The listing builds one solid part. Answer for the finished solid, in the listing's coordinates (mm). A direction names the side the tool comes from. Give positions to 0.01 mm unless a question says otherwise; leave off trailing zeros. Order: outer loops, then holes, each group sorted by start corner. A loop starts at its lowest first (then second) coordinate and runs counter-clockwise, first axis right, second up. Notation, with made-up numbers: (59.25, 3) -> (86.25, 3) arc R20 cw to (86.25, 15) -> close; hole circle Ø1 at (6, 52.25). An arc over 180 degrees is marked (long way). Write item = value, one per line. Start each with the question number.
```python
from build123d import *

# Parameters (mm, degrees)
SKETCH1_R                     = 36.6395
HOUSING_FITTING_EXTRUDE_DEPTH = 16.637
HOUSING_BODY_1_DEPTH          = 21.2725
SKETCH3_R                     = 6.731
IMPELLER_BORE_DEPTH           = 17.018
SKETCH4_R                     = 4
SHAFT_BORE_DEPTH              = 20.8915
O_RING_CUT_DEPTH              = 1.27
O_RING_CUT_DEPTH_BACK         = 3.175
SKETCH5_R                     = 36.6395
SKETCH5_R_2                   = 34.2265
SKETCH12_R                    = 3.175
CUT_EXTRUDE2_DEPTH            = 21.2725
CIRPATTERN1_COUNT             = 8
SKETCH13_R                    = 3.175
CUT_EXTRUDE3_DEPTH            = 16.51
SKETCH14_R                    = 3.175
SKETCH14_R_2                  = 3.392842108
CUT_EXTRUDE4_DEPTH            = 16.51
SKETCH15_R                    = 3.175
CUT_EXTRUDE5_DEPTH            = 10.922
FILLET1_R                     = 6.604
SKETCH17_R                    = 17.5006
CUT_EXTRUDE8_DEPTH            = 25.2095
BOSS_EXTRUDE1_START           = 6.35
SKETCH18_R                    = 17.5006
SKETCH18_R_2                  = 15.875
BOSS_EXTRUDE1_DEPTH           = 6.35


with BuildPart() as part:
    # Sketch1 → Housing Fitting Extrude (new body)
    with BuildSketch(Plane(origin=(0, 0, 0), x_dir=(0, 0, -1), z_dir=(1, 0, 0))):
        Circle(SKETCH1_R)
    extrude(amount=HOUSING_FITTING_EXTRUDE_DEPTH)

    # Sketch2 → Housing Body 1 (add)
    with BuildSketch(Plane.ZY):
        with BuildLine():
            Line((60.96, 0), (60.96, 60.96))
            Line((60.96, 60.96), (0, 60.96))
            ThreePointArc((0, 60.96), (-43.105229381, 43.105229381), (-60.96, 0))
            Line((-60.96, 0), (-60.96, -54.61))
            Line((-60.96, -54.61), (-60.96, -60.96))
            Line((-60.96, -60.96), (60.96, -60.96))
            Line((60.96, -60.96), (60.96, -54.61))
            Line((60.96, -54.61), (60.96, 0))
        make_face()
    extrude(amount=HOUSING_BODY_1_DEPTH)

    # Sketch3 → Impeller Bore (cut)
    with BuildSketch(Plane(origin=(16.637, 0, 0), x_dir=(0, 0, -1), z_dir=(1, 0, 0))):
        Circle(SKETCH3_R)
    extrude(amount=-IMPELLER_BORE_DEPTH, mode=Mode.SUBTRACT)

    # Sketch4 → Shaft Bore (cut)
    with BuildSketch(Plane(origin=(-0.381, 0, 0), x_dir=(0, 0, -1), z_dir=(1, 0, 0))):
        Circle(SKETCH4_R)
    extrude(amount=-SHAFT_BORE_DEPTH, mode=Mode.SUBTRACT)

    # Sketch5 → O-Ring Cut (cut, two sides: drawn at the far end of the back side and taken through both)
    with BuildSketch(Plane(origin=(8.509, 0, 0), x_dir=(0, 0, -1), z_dir=(1, 0, 0)).offset(-O_RING_CUT_DEPTH_BACK)):
        Circle(SKETCH5_R)
        Circle(SKETCH5_R_2, mode=Mode.SUBTRACT)
    extrude(amount=O_RING_CUT_DEPTH + O_RING_CUT_DEPTH_BACK, mode=Mode.SUBTRACT)

    # Sketch12 → Cut-Extrude2 (cut)
    with BuildSketch(Plane(origin=(0, 0, 0), x_dir=(0, 0, -1), z_dir=(1, 0, 0))):
        with Locations((-50.8, 0)):
            Circle(SKETCH12_R)
    cut_extrude2 = extrude(amount=-CUT_EXTRUDE2_DEPTH, mode=Mode.SUBTRACT)

    # CirPattern1: Cut-Extrude2 ×8 about axis, 1 skipped
    cirpattern1_axis = Axis((0, 0, 0), (1, 0, 0))
    add([cut_extrude2.rotate(cirpattern1_axis, i * 360 / CIRPATTERN1_COUNT) for i in range(1, CIRPATTERN1_COUNT) if i not in (7,)], mode=Mode.SUBTRACT)

    # Sketch13 → Cut-Extrude3 (cut)
    with BuildSketch(Plane.XY.offset(60.96)):
        with Locations((-9.525, -41.817738443)):
            Circle(SKETCH13_R)
    extrude(amount=-CUT_EXTRUDE3_DEPTH, mode=Mode.SUBTRACT)

    # Sketch14 → Cut-Extrude4 (cut)
    with BuildSketch(Plane.XZ.offset(60.96)):
        with Locations(Location((-9.525, -46.754349092, 0), (0, 0, 270))):
            Circle(SKETCH14_R)
        with Locations(Location((-9.525, 41.914080666, 0), (0, 0, 270))):
            Circle(SKETCH14_R_2)
    extrude(amount=-CUT_EXTRUDE4_DEPTH, mode=Mode.SUBTRACT)

    # Sketch15 → Cut-Extrude5 (cut)
    with BuildSketch(Plane(origin=(0, 0, -60.96), x_dir=(-1, 0, 0), z_dir=(0, 0, -1))):
        with Locations(Location((9.525, -39.337514031, 0), (0, 0, 90))):
            Circle(SKETCH15_R)
    extrude(amount=-CUT_EXTRUDE5_DEPTH, mode=Mode.SUBTRACT)

    # Fillet1
    fillet1_edges = [part.edges().sort_by_distance(p)[0] for p in [
        (16.637, 0, 6.731),
    ]]
    fillet(fillet1_edges, radius=FILLET1_R)

    # Sketch17 → Cut-Extrude8 (cut)
    with BuildSketch(Plane.ZY.offset(21.2725)):
        Circle(SKETCH17_R)
    extrude(amount=-CUT_EXTRUDE8_DEPTH, mode=Mode.SUBTRACT)

    # Sketch18 → Boss-Extrude1 (add)
    with BuildSketch(Plane.ZY.offset(-3.937).offset(BOSS_EXTRUDE1_START)):
        Circle(SKETCH18_R)
        Circle(SKETCH18_R_2, mode=Mode.SUBTRACT)
    extrude(amount=-BOSS_EXTRUDE1_DEPTH)


solid = part.part
```
Item 1: A cutting plane is placed at A-A, the plane y = -50.8. Count the separate pieces of the cut face and the enclosed holes in it, plus the area to 3 significant figures.
Item 2: A cutting plane is placed at C-C, the plane y = 50.8. Write down the section's boundary in (x, z) (1 decimal), plus the area to 3 significant figures.
Item 3: Which of the six approach directions +Z, -Z, +X, -X, +Y, -Y give full straight-line access (tool end or side, diameter ignored) to faces 5 (the flat face through (0, -26.2, 26.2)), 6 (the cylindrical face through (-10.21, -44.92, 52.82)), 7 (the cylindrical face through (-10.49, -53.97, 0.14)), 8 (the flat face through (3.937, 0, 7))?
Item 4: Flat-ended cylindrical pins translate along their axes: pin 1 (4 mm diameter, centred on y = -40.5, z = -24, fed in from +X); pin 2 (8.5 mm diameter, centred on x = -9.52, y = -41.82, fed in from -Z); pin 3 (3 mm diameter, centred on x = -9, y = -40.5, fed in from +Z); pin 4 (1.5 mm diameter, centred on x = 9.5, y = -30.5, fed in from -Z). Find the tip coordinate at first contact, or state that the pin passes through.
Item 5: The mould has two halves that part along Z. Classify faces 1 (the flat face through (5.334, 33, 11)), 2 (the flat face through (-9, -39, -50.038)), 3 (the cylindrical face through (13.16, 11.006, -34.948)), 4 (the cylindrical face through (-10.49, -38.44, -33.99)): +Z half, -Z half, draft (parallel to the pull), parting line (faces both ways), or undercut.
Item 6: Consider L1, parallel to Y at x = 0.75, z = 0 (1 decimal); L2, parallel to X at y = -7, z = -34; L3, parallel to Y at x = 9.5, z = 0.5. Determine where each line is inside the solid, lowest interval first. Write a range as from..to.
Item 7: A cutting plane is placed at D-D, the plane z = 23. Write down the section's boundary in (x, y), plus the area to 3 significant figures.
Check values:
q1.separate_pieces = 2
q1.enclosed_holes = 2
q1.area = 2,390 mm^2
q2.outline = (-21.3, -33.7) -> (0, -33.7) -> (0, -3.2) -> (-21.3, -3.2) -> close; (-21.3, 3.2) -> (0, 3.2) -> (0, 61) -> (-21.3, 61) -> close
q2.area = 1,880 mm^2
q3.face_5 = +X
q3.face_6 = +Z
q3.face_7 = +X, -X
q3.face_8 = -X
q4.pin_1 = 0
q4.pin_2 = -60.96
q4.pin_3 = 44.45
q4.pin_4 = -21.31
q5.face_1 = draft
q5.face_2 = -Z half
q5.face_3 = parting line
q5.face_4 = undercut
q6.L1 = -36.6..-15.9, 15.9..36.6
q6.L2 = -21.27..5.33, 9.78..16.64
q6.L3 = -34.22..-6.71, 6.71..34.22
q7.outline = (-21.27, -60.96) -> (0, -60.96) -> (0, -28.52) -> (5.33, -28.52) -> (5.33, -25.35) -> (9.78, -25.35) -> (9.78, -28.52) -> (16.64, -28.52) -> (16.64, 28.52) -> (9.78, 28.52) -> (9.78, 25.35) -> (5.33, 25.35) -> (5.33, 28.52) -> (0, 28.52) -> (0, 60.96) -> (-21.27, 60.96) -> close
q7.area = 3,510 mm^2
